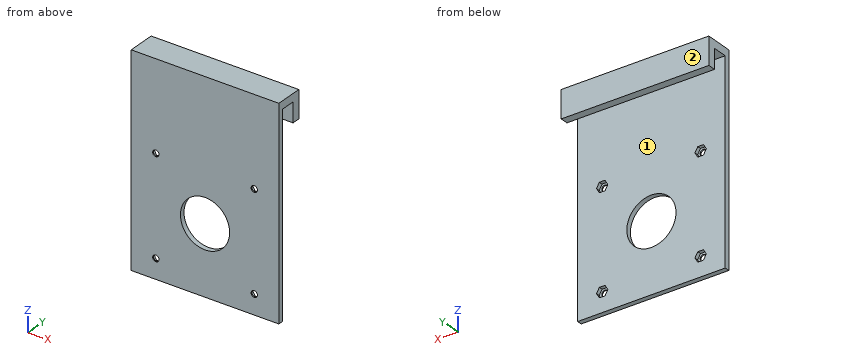
Autodesk Inventor part; units mm, degrees
ref_plane "YZ Plane" through (0, 0, 0) normal (1, 0, 0) x (0, 1, 0)
ref_plane "XZ Plane" through (0, 0, 0) normal (0, 1, 0) x (-1, 0, 0)
ref_plane "XY Plane" through (0, 0, 0) normal (0, 0, 1) x (1, 0, 0)
sketch "Sketch1" plane through (0, 0, 0) normal (0, 1, 0) x (-1, 0, 0)
  line L0 (0, 0) -> (150, 0)
  line L1 (150, 0) -> (150, -210)
  line L2 (150, -210) -> (0, -210)
  line L3 (0, -210) -> (0, 0)
  dimension "d11" = 150
  dimension "d12" = 210
extrude "Extrusion1" add sketch "Sketch1" along normal blind 5
sketch "Sketch2" plane through (0, 5, 0) normal (0, 1, 0) x (1, 0, 0)
  line L0 (-150, 0) -> (0, 0)
  line L1 (-150, 210) -> (-150, 0)
  line L2 (0, 0) -> (-150, 0)
  line L3 (-150, 0) -> (-150, 8)
  line L4 (-150, 8) -> (0, 8)
  line L5 (0, 8) -> (0, 0)
  dimension "d13" = 8
extrude "Extrusion2" add sketch "Sketch2" along normal blind 23
sketch "Sketch3" plane through (0, 5, -8) normal (0, 0, -1) x (-1, 0, 0)
  line L0 (150, 23) -> (0, 23)
  line L1 (150, -5) -> (150, 23)
  line L2 (0, 23) -> (150, 23)
  line L3 (150, 23) -> (150, 15)
  line L4 (150, 15) -> (0, 15)
  line L5 (0, 15) -> (0, 23)
  point P0 (0, -5)
  dimension "d14" = 8
extrude "Extrusion3" add sketch "Sketch3" along normal blind 20
sketch "Sketch6" plane through (0, 5, 0) normal (0, 1, 0) x (1, 0, 0)
  line L0 (-150, 8) -> (0, 8)
  line L1 (-75, 8) -> (-75, 210)
  line L2 (0, 210) -> (-150, 210)
  line L3 (-150, 210) -> (-150, 8)
  line L4 (-150, 140) -> (0, 140)
  line L5 (0, 8) -> (0, 210)
  circle A0 centre (-125, 90) radius 3.2
  circle A1 centre (-125, 190) radius 3.2
  circle A2 centre (-25, 190) radius 3.2
  circle A3 centre (-25, 90) radius 3.2
  line L6 (-150, 0) -> (0, 0)
  dimension "d44" = 50
  dimension "d45" = 6.4
  dimension "d46" = 50
  dimension "d64" = 140
hole "Hole2" at (-25, 5, -190) at (-25, 5, -90) at (-125, 5, -90) at (-125, 5, -190) direction (0, -1, 0) diameter 6.4 end through all counterbore diameter 9 counterbore depth 3.8
sketch "Sketch5" plane through (0, 5, 0) normal (0, 1, 0) x (1, 0, 0)
  line L0 (-27.8868, 195) -> (-22.1132, 195)
  line L1 (-22.1132, 195) -> (-19.2265, 190)
  line L2 (-19.2265, 190) -> (-22.1132, 185)
  line L3 (-22.1132, 185) -> (-27.8868, 185)
  line L4 (-27.8868, 185) -> (-30.7735, 190)
  line L5 (-30.7735, 190) -> (-27.8868, 195)
  line L6 (-27.8868, 85) -> (-30.7735, 90)
  line L7 (-30.7735, 90) -> (-27.8868, 95)
  line L8 (-27.8868, 95) -> (-22.1132, 95)
  line L9 (-22.1132, 95) -> (-19.2265, 90)
  line L10 (-19.2265, 90) -> (-22.1132, 85)
  line L11 (-22.1132, 85) -> (-27.8868, 85)
  line L12 (-127.8868, 185) -> (-130.7735, 190)
  line L13 (-130.7735, 190) -> (-127.8868, 195)
  line L14 (-127.8868, 195) -> (-122.1132, 195)
  line L15 (-122.1132, 195) -> (-119.2265, 190)
  line L16 (-119.2265, 190) -> (-122.1132, 185)
  line L17 (-122.1132, 185) -> (-127.8868, 185)
  line L18 (-150, 210) -> (0, 210)
  line L19 (-75, 210) -> (-75, 30.6019)
  line L20 (-127.8868, 85) -> (-130.7735, 90)
  line L21 (-130.7735, 90) -> (-127.8868, 95)
  line L22 (-127.8868, 95) -> (-122.1132, 95)
  line L23 (-122.1132, 95) -> (-119.2265, 90)
  line L24 (-119.2265, 90) -> (-122.1132, 85)
  line L25 (-122.1132, 85) -> (-127.8868, 85)
  line L26 (-150, 210) -> (-150, 8)
  line L27 (-146.8054, 140) -> (0, 140)
  line L28 (0, 210) -> (0, 0)
  line L29 (-150, 0) -> (0, 0)
  point P0 (-25, 190)
  point P1 (-25, 90)
  point P2 (-125, 190)
  point P3 (-125, 90)
  dimension "d34" = 10
  dimension "d54" = 10
  dimension "d55" = 10
  dimension "d56" = 10
  dimension "d57" = 100
  dimension "d58" = 100
  dimension "d65" = 140
extrude "Extrusion6" cut sketch "Sketch5" against normal blind 3.8 contours L0 L1 L2 L3 L4 L5 | L6 L7 L8 L9 L10 L11 | L12 L13 L14 L15 L16 L17 | L20 L21 L22 L23 L24 L25
sketch "Sketch7" plane through (0, 5, 0) normal (0, 1, 0) x (1, 0, 0)
  circle A0 centre (-75, 140) radius 27.9443
  line L0 (-150, 140) -> (0, 140)
  line L1 (-150, 210) -> (0, 210)
  line L2 (-75, 210) -> (-75, 0)
  line L3 (0, 210) -> (0, 0)
  line L4 (-150, 210) -> (0, 210)
  line L5 (0, 210) -> (0, 0)
  line L6 (0, 0) -> (-150, 0)
  line L7 (-150, 0) -> (-150, 210)
  line L8 (0, 8) -> (0, 210)
  line L9 (-150, 210) -> (-150, 8)
  line L10 (0, 210) -> (-150, 210)
  line L11 (-150, 0) -> (0, 0)
  dimension "d66" = 140
hole "Hole3" at (-75, 5, -140) direction (0, -1, 0) diameter 50 end through all
properties part number "Stand"
Work out the finished part from the listing and answer in its coordinate system (mm). Face numbers are marked on the shaded views. A direction names the side the tool comes from. Give positions to 0.01 mm unless a question says otherwise; leave off trailing zeros. Write each loop counter-clockwise with the first axis right and the second up, starting at its lowest first coordinate (ties: lowest second). Pieces come first, ordered by that corner, then holes.
Q1. A tool of negligible diameter and unlimited length cuts with its end or side. For the marked faces 1 and 2, from which of +Z, -Z, +X, -X, +Y, -Y can it reach the whole face along a straight path? Write none if from no direction.
Answer:
face 1: -Z, +X, -X
face 2: +Z, -Z, +X, -X, +Y
Q2. Given pin 1 (3 mm diameter, centred on x = -127.5, z = -189.5, fed in from +Y); pin 2 (8 mm diameter, centred on x = -29, y = 10.5, fed in from -Z); pin 3 (5 mm diameter, centred on x = -28, z = -90, fed in from +Y); pin 4 (6 mm diameter, centred on x = -25, z = -90, fed in from -Y), each flat-ended and moving along its own axis, determine where each tip first touches the part or whether it passes through.
Answer:
pin 1: stops at y = 1.2
pin 2: stops at z = -8
pin 3: stops at y = 5
pin 4: passes through
Q3. The part is cut by section A-A on z = -140. Give the vertices of the cut face in (x, y), and give its area (3 significant figures).
Answer:
outline: (-150, 0) - (-100, 0) - (-100, 5) - (-150, 5) - close; (-50, 0) - (0, 0) - (0, 5) - (-50, 5) - close
area: 500 mm2
Q4. The part is cut by section C-C on x = -109.5. Give the vertices of the cut face in (y, z).
Answer:
outline: (0, -210) - (5, -210) - (5, -8) - (20, -8) - (20, -28) - (28, -28) - (28, 0) - (0, 0) - close
Q5. The part is cut by section B-B on x = -25. Give the vertices of the cut face in (y, z), and give its area (3 significant figures).
Answer:
outline: (0, -210) - (5, -210) - (5, -195) - (1.2, -195) - (1.2, -193.2) - (0, -193.2) - close; (0, -186.8) - (1.2, -186.8) - (1.2, -185) - (5, -185) - (5, -95) - (1.2, -95) - (1.2, -93.2) - (0, -93.2) - close; (0, -86.8) - (1.2, -86.8) - (1.2, -85) - (5, -85) - (5, -8) - (20, -8) - (20, -28) - (28, -28) - (28, 0) - (0, 0) - close
area: 1,300 mm2
Q6. The part is cut by section D-D on x = -67. Give the vertices of the cut face in (y, z), and give its area (3 significant figures).
Answer:
outline: (0, -210) - (5, -210) - (5, -163.69) - (0, -163.69) - close; (0, -116.31) - (5, -116.31) - (5, -8) - (20, -8) - (20, -28) - (28, -28) - (28, 0) - (0, 0) - close
area: 1,160 mm2
Q7. Straight lines are drawn through the part: L1, parallel to X at y = 0.9, z = -90; L2, parallel to Z at x = -125, y = 0.45; L3, parallel to Y at x = -82, z = -171. For each, find the intervals that lie inside material, in ascending order.
Answer:
L1: x = -150 to -128.2, -121.8 to -28.2, -21.8 to 0
L2: z = -210 to -193.2, -186.8 to -93.2, -86.8 to 0
L3: y = 0 to 5
